```python
from build123d import *

# Parameters (mm, degrees)
SKETCH3_W                = 44.5
SKETCH3_H                = 44
SKETCH3_R                = 13.462
SKETCH3_R_2              = 1.554126588
FRONT_FACE_DEPTH         = 5
SKETCH4_W                = 44.5
SKETCH4_H                = 54
BOTTOM_PLATE_DEPTH       = 2
RIB_DEPTH                = 0.5
SKETCH6_W                = 6.5
SKETCH6_H                = 54
SKETCH6_R                = 1.5
BOTTOM_SCREW_HOLES_DEPTH = 2
SKETCH7_W                = 43.5
SKETCH7_H                = 3
CUT_EXTRUDE1_DEPTH       = 44
SKETCH8_R                = 3.554126588
SKETCH8_R_2              = 1.554126588
BOSS_EXTRUDE5_DEPTH      = 3


with BuildPart() as part:
    # Sketch3 → Front Face (new body)
    with BuildSketch(Plane.XZ):
        with Locations((0, -22)):
            Rectangle(SKETCH3_W, SKETCH3_H)
        with Locations((0, -21.209)):
            Circle(SKETCH3_R, mode=Mode.SUBTRACT)
        with Locations((15.494, -5.715)):
            Circle(SKETCH3_R_2, mode=Mode.SUBTRACT)
        with Locations((-15.494, -5.715)):
            Circle(SKETCH3_R_2, mode=Mode.SUBTRACT)
        with Locations((-15.494, -36.703)):
            Circle(SKETCH3_R_2, mode=Mode.SUBTRACT)
        with Locations((15.494, -36.703)):
            Circle(SKETCH3_R_2, mode=Mode.SUBTRACT)
    front_face = extrude(amount=FRONT_FACE_DEPTH)

    # Sketch4 → Bottom Plate (add)
    with BuildSketch(Plane.XY):
        with Locations((0, 22)):
            Rectangle(SKETCH4_W, SKETCH4_H)
    bottom_plate = extrude(amount=BOTTOM_PLATE_DEPTH)

    # Sketch5 → Rib (add)
    with BuildSketch(Plane.ZY.offset(22.25)):
        Polygon((-21.209, 0), (0, 21.209), (0, 0), align=None)
    rib = extrude(amount=-RIB_DEPTH)

    # Sketch6 → Bottom Screw Holes (add)
    with BuildSketch(Plane(origin=(21.209, 47.45, 0), x_dir=(-1, 0, 0), z_dir=(0, 0, -1))):
        with Locations((46.709, -25.45)):
            Rectangle(SKETCH6_W, SKETCH6_H)
        with Locations((46.709, -49.45)):
            Circle(SKETCH6_R, mode=Mode.SUBTRACT)
        with BuildLine():
            Line((48.209, -2.95), (48.209, -27.95))
            ThreePointArc((48.209, -27.95), (46.709, -29.45), (45.209, -27.95))
            Line((45.209, -27.95), (45.209, -2.95))
            ThreePointArc((45.209, -2.95), (46.709, -1.45), (48.209, -2.95))
        make_face(mode=Mode.SUBTRACT)
    bottom_screw_holes = extrude(amount=-BOTTOM_SCREW_HOLES_DEPTH)

    # Mirror of Rib and Bottom Screws: Front Face, Bottom Plate, Rib, Bottom Screw Holes across plane
    add(front_face.mirror(Plane.ZY))
    add(bottom_plate.mirror(Plane.ZY))
    add(rib.mirror(Plane.ZY))
    add(bottom_screw_holes.mirror(Plane.ZY))

    # Sketch7 → Cut-Extrude1 (cut)
    with BuildSketch(Plane(origin=(0, 0, -44), x_dir=(-1, 0, 0), z_dir=(0, 0, -1))):
        with Locations((0, -1.5)):
            Rectangle(SKETCH7_W, SKETCH7_H)
    extrude(amount=-CUT_EXTRUDE1_DEPTH, mode=Mode.SUBTRACT)

    # Sketch8 → Boss-Extrude5 (add)
    with BuildSketch(Plane(origin=(0, -3, 0), x_dir=(1, 0, 0), z_dir=(0, 1, 0))):
        with Locations((-15.494, 36.703)):
            Circle(SKETCH8_R)
        with Locations((-15.494, 36.703)):
            Circle(SKETCH8_R_2, mode=Mode.SUBTRACT)
        with Locations((15.494, 36.703)):
            Circle(SKETCH8_R)
        with Locations((15.494, 36.703)):
            Circle(SKETCH8_R_2, mode=Mode.SUBTRACT)
        with Locations((15.494, 5.715)):
            Circle(SKETCH8_R)
        with Locations((15.494, 5.715)):
            Circle(SKETCH8_R_2, mode=Mode.SUBTRACT)
        with Locations((-15.494, 5.715)):
            Circle(SKETCH8_R)
        with Locations((-15.494, 5.715)):
            Circle(SKETCH8_R_2, mode=Mode.SUBTRACT)
    extrude(amount=BOSS_EXTRUDE5_DEPTH)


solid = part.part
```
Design review of the part built by this model. Coordinates are the model's own, in mm. A direction names the side the tool comes from. Coordinates: 2 decimals unless noted, no trailing zeros. Loops run counter-clockwise (first coordinate to the right, second up) from the corner with the lowest first, then second, coordinate; pieces in that order, holes last.
Q1. The part is to be moulded in two halves that separate along Y. For faces 1 (the face through (-25.5, 18, 1)), 2 (the face through (13.94, -2.46, -5.65)), 3 (the face through (-27, 32, 1)), 4 (the face through (0, 49, 1)), say which applies: +Y half, -Y half, draft (parallel to the pull), parting line (faces both ways), or undercut.
Reported:
face 1: undercut
face 2: draft
face 3: undercut
face 4: +Y half
Q2. We need section B-B on x = -25.5. State the section outline as (y, z) points.
Reported:
outline: (-5, 0) - (-3.5, 0) - (-3.5, 2) - (-5, 2) - close; (-0.5, 0) - (18, 0) - (18, 2) - (-0.5, 2) - close; (46, 0) - (49, 0) - (49, 2) - (46, 2) - close
Q3. Tool access review of faces 5 (the face through (24, 32, 1)), 6 (the face through (-15, 0, -35)), 7 (the face through (-22.25, 2, -17)), 8 (the face through (10, -3, -32)): name each direction out of +Z, -Z, +X, -X, +Y, -Y from which nothing blocks a thin tool from reaching the whole face with its end or side.
Reported:
face 5: +Z, -Z
face 6: -Z, +X, -X, +Y
face 7: -Z, -X, +Y, -Y
face 8: +Y
Q4. To check wall thickness, follow line 1 (Z direction, x = 0, y = -3.55); line 2 (X direction, y = -1.5, z = -9); line 3 (X direction, y = 14, z = -4). State the ranges of each line that lie inside material, in increasing order.
Reported:
line 1: z = -44 to -34.67, -7.75 to 2
line 2: x = -22.25 to -21.75, -16.85 to -14.14, 14.14 to 16.85, 21.75 to 22.25
line 3: x = -22.25 to -21.75, 21.75 to 22.25
Q5. We need section A-A on y = 28. State the section outline as (x, z) points.
Reported:
outline: (-28.75, 0) - (-27, 0) - (-27, 2) - (-28.75, 2) - close; (-24, 0) - (24, 0) - (24, 2) - (-24, 2) - close; (27, 0) - (28.75, 0) - (28.75, 2) - (27, 2) - close
Q6. We need section C-C on y = -2. State how many separate pieces and enclosed holes the cut face has, and give its area (3 significant figures).
Reported:
separate pieces: 7
enclosed holes: 4
area: 275 mm2
Q7. We need section D-D on z = -30. State the section outline as (x, y) points, and give its area (3 significant figures).
Reported:
outline: (-22.25, -5) - (-10.2, -5) - (-10.2, -3) - (-21.75, -3) - (-21.75, 0) - (-22.25, 0) - close; (10.2, -5) - (22.25, -5) - (22.25, 0) - (21.75, 0) - (21.75, -3) - (10.2, -3) - close
area: 51.2 mm2
Q8. For pin 1 (3.5 mm diameter, centred on x = 14.5, z = -36, fed in from +Y); pin 2 (2 mm diameter, centred on y = 16.5, z = -2.5, fed in from +X); pin 3 (5 mm diameter, centred on x = -15.494, z = -5.715, fed in from -Y); pin 4 (4 mm diameter, centred on x = 12, y = 30.5, fed in from -Z), all flat-tipped, find the tip position at first contact; note any pin that passes through.
Reported:
pin 1: stops at y = 0
pin 2: stops at x = 22.25
pin 3: stops at y = -5
pin 4: stops at z = 0
